Part model, mm, in its own coordinate system. A direction names the side the tool comes from. Round coordinates to 2 decimals unless told otherwise and drop trailing zeros. Write each loop counter-clockwise with the first axis right and the second up, starting at its lowest first coordinate (ties: lowest second). Pieces come first, ordered by that corner, then holes. Notation, with made-up numbers: M -1,15 L 40,15 A25 cw 40,53 Z; hole C 53,59 d9. An arc over 180 degrees is marked long. Use a Markdown table: item, result. Add a question column.
1) Which spindle directions (+Z, -Z, +X, -X, +Y, -Y) get a long thin tool onto all of the face, cutting with end or side? Do faces 1 (the face through (1362, 343, -680)), 2 (the face through (-563.134, 344, -361)), 3 (the face through (382, -304.061, -36)). Say none if no direction does.
2) Drop a flat-ended pin along its axis: P1, Ø8, axis at x = 913, y = 8.5, coming from the -Z side. Give the stop position or say it passes through.
3) Slice it at B-B on y = -52. Write the cut outline in (x, z).
4) Two-plate mould, pull along Y, no slides. Class faces 4 (the face through (374, 343, -50)), 5 (the face through (-579.888, 15, -25)), 6 (the face through (382, -339.061, -39)): released by +Y, released by -Y, zero draft, split by the parting line, or undercut.
5) Wall check: probe 1 along Z at (x, y) = (-312, -167); probe 2 along X at (y, z) = (-310, -430); probe 3 along Z at (x, y) = (1155, 329.5). Give the ranges that are in metal, low to high.
6) Slice it at C-C on x = 1143. Write the cut outline in (y, z).
7) Slice it at A-A on z = -85.5. Write the cut outline in (x, y).
```python
from build123d import *

# Parameters (mm, degrees)
F0_W     = 2000
F0_H     = 700
F1_DEPTH = 25
F3_DEPTH = 50
F5_W     = 50
F5_H     = 35
F6_DEPTH = 630


with BuildPart() as f1:
    # F0 (on Top) → F1 (new body)
    with BuildSketch(Plane.XY):
        with Locations((386.865544, 10.939363)):
            Rectangle(F0_W, F0_H)
    extrude(amount=F1_DEPTH)

    # F2 (on face) → F3 (join)
    with BuildSketch(Plane(origin=(0, 0, 0), x_dir=(1, 0, 0), z_dir=(0, 0, -1))):
        Polygon((-613.134456, -360.939363), (1052.856326, -360.939363), (1052.856326, -325.939363), (-579.887948, -325.939363), (-579.887948, 0), (-613.134456, -10.939363), align=None)
        Polygon((1052.856326, -325.939363), (1052.856326, -360.939363), (1386.865544, -360.939363), (1386.865544, -10.939363), (1351.865544, -10.939363), (1351.865544, -325.939363), align=None)
        Polygon((1351.865544, -10.939363), (1386.865544, -10.939363), (1386.865544, 339.060637), (1052.856326, 339.060637), (1052.856326, 304.060637), (1351.865544, 304.060637), align=None)
        Polygon((-613.134456, 339.060637), (-613.134456, -10.939363), (-579.887948, 0), (-579.887948, 304.060637), (1052.856326, 304.060637), (1052.856326, 339.060637), align=None)
    extrude(amount=F3_DEPTH)

    # F5 (on face) → F6 (join)
    with BuildSketch(Plane(origin=(0, 0, -50), x_dir=(1, 0, 0), z_dir=(0, 0, -1))):
        with Locations((-588.134456, 321.560637)):
            Rectangle(F5_W, F5_H)
        with Locations((-588.134456, -343.439363)):
            Rectangle(F5_W, F5_H)
        with Locations((1361.865544, -343.439363)):
            Rectangle(F5_W, F5_H)
        with Locations((1361.865544, 321.560637)):
            Rectangle(F5_W, F5_H)
    extrude(amount=F6_DEPTH)


solid = f1.part
```
Entries:
| question | item | result |
|---|---|---|
| 1 | face 1 | -Z, +X, -X, +Y, -Y |
| 1 | face 2 | -Z, +Y, -Y |
| 1 | face 3 | -Z |
| 2 | P1 | stops at z = 0 |
| 3 | outline | M -613.13,-50 L -579.89,-50 L -579.89,0 L 1351.87,0 L 1351.87,-50 L 1386.87,-50 L 1386.87,25 L -613.13,25 Z |
| 4 | face 4 | zero draft |
| 4 | face 5 | undercut |
| 4 | face 6 | released by -Y |
| 5 | probe 1 | z = 0 to 25 |
| 5 | probe 2 | x = -613.13 to -563.13, 1336.87 to 1386.87 |
| 5 | probe 3 | z = -50 to 25 |
| 6 | outline | M -339.06,-50 L -304.06,-50 L -304.06,0 L 325.94,0 L 325.94,-50 L 360.94,-50 L 360.94,25 L -339.06,25 Z |
| 7 | outline | M -613.13,-339.06 L -563.13,-339.06 L -563.13,-304.06 L -613.13,-304.06 Z; M -613.13,325.94 L -563.13,325.94 L -563.13,360.94 L -613.13,360.94 Z; M 1336.87,-339.06 L 1386.87,-339.06 L 1386.87,-304.06 L 1336.87,-304.06 Z; M 1336.87,325.94 L 1386.87,325.94 L 1386.87,360.94 L 1336.87,360.94 Z |
